Answer from the drawing. Dimensions are ordinates in mm from the lowest x, y and z of the part. A direction names the side the tool comes from. Coordinates: 2 decimals unless noted, no trailing zeros. Write each loop counter-clockwise with the first axis right and the second up, starting at its lowest first coordinate (ties: lowest second). Pieces come first, ordered by that corner, then holes.
(1) The part is cut by section A-A on z = 92. Determine the outline of the cut face in (x, y).
(2) The part is cut by section D-D on x = 36.5. Determine the outline of the cut face in (y, z) (1 decimal).
(3) The part is cut by section B-B on y = 11.25. Determine the outline of the cut face in (x, z) (1 decimal), plus the area to 3 significant figures.
(4) Which of the six approach directions +Z, -Z, +X, -X, +Y, -Y give full straight-line access (tool end or side, diameter ignored) to the marked faces 1, 2 and 3?
(5) Straight lines are drawn through the part: line 1 (X direction, y = 3.25, z = 111.5) (1 decimal); line 2 (X direction, y = 1.5, z = 109.5) (1 decimal); line 3 (X direction, y = 21, z = 47.5). For each, find the intervals that lie inside material, in ascending order.
(6) Given P1, Ø6, axis at x = 37.5, y = 5.5, coming from the -Z side; P2, Ø12, axis at y = 14, z = 109, coming from the -X side; P3, Ø7.5, axis at x = 101, y = 7.5, coming from the +Z side; P4, Ø1.5, axis at y = 10.5, z = 94.5, coming from the -X side, each flat-ended and moving along its own axis, determine where each tip first touches the part or whether it passes through.
(7) For a pull along Z with two mould halves and no side action, classify the marked faces 4, 5 and 6 as +Z half, -Z half, draft (parallel to the pull), parting line (faces both ways), or undercut.
(8) The part is cut by section C-C on x = 88. Determine the outline of the cut face in (y, z) (1 decimal).
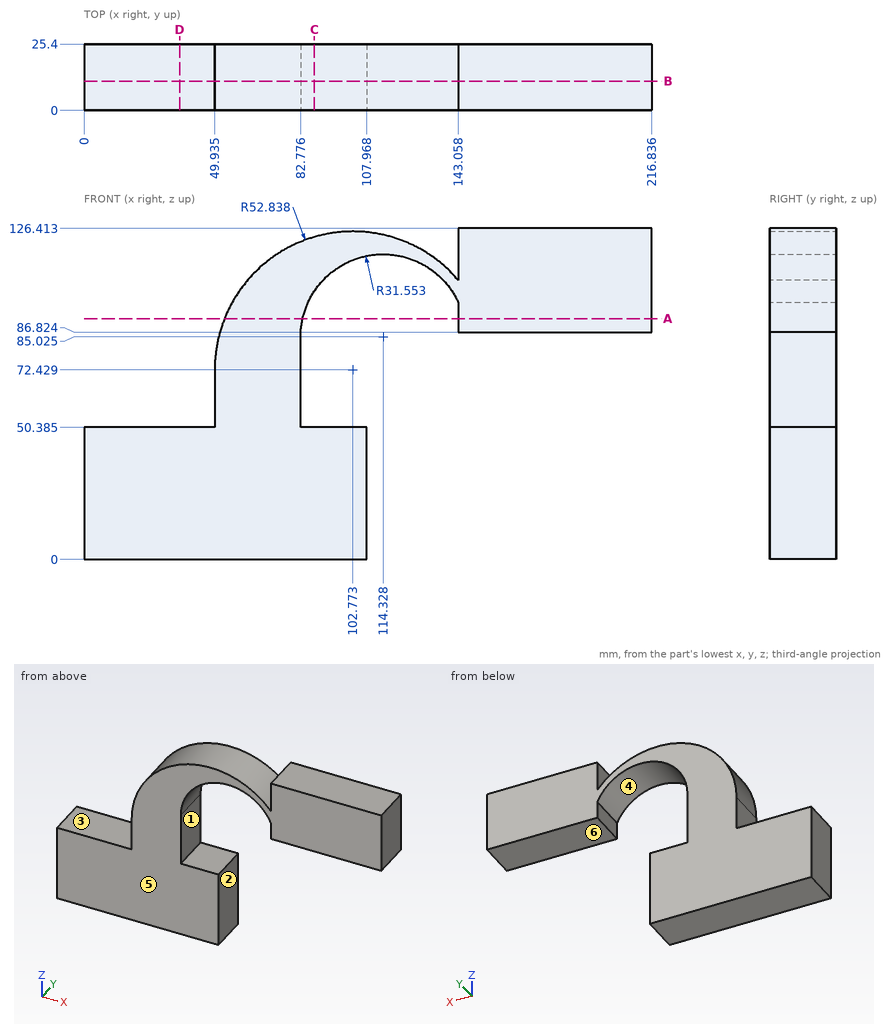
Model answer:
1. outline: (53.69, 0) - (83.56, 0) - (83.56, 25.4) - (53.69, 25.4) - close; (143.06, 0) - (216.84, 0) - (216.84, 25.4) - (143.06, 25.4) - close
2. outline: (0, 0) - (25.4, 0) - (25.4, 50.4) - (0, 50.4) - close
3. outline: (0, 0) - (108, 0) - (108, 50.4) - (82.8, 50.4) - (82.8, 85) arc R31.6 cw to (143.1, 98.1) - (143.1, 86.8) - (216.8, 86.8) - (216.8, 126.4) - (143.1, 126.4) - (143.1, 106.6) arc R52.8 ccw to (49.9, 72.4) - (49.9, 50.4) - (0, 50.4) - close
3. area: 10,900 mm2
4. face 1: +X, +Y, -Y
4. face 2: -Z, +X, +Y, -Y
4. face 3: +Z, -X, +Y, -Y
5. line 1: x = 67.2 to 97.2, 131.5 to 138.3, 143.1 to 216.8
5. line 2: x = 65.1 to 94.4, 134.2 to 140.4, 143.1 to 216.8
5. line 3: x = 0 to 107.97
6. P1: stops at z = 0
6. P2: stops at x = 59.68
6. P3: stops at z = 125.27
6. P4: stops at x = 54.43
7. face 4: undercut
7. face 5: draft
7. face 6: -Z half
8. outline: (0, 0) - (25.4, 0) - (25.4, 50.4) - (0, 50.4) - close; (0, 102.4) - (25.4, 102.4) - (25.4, 123.2) - (0, 123.2) - close
